Input: dimensioned drawing with shaded views. Units: mm. Origin: part minimum x, y, z. Give positions to 0.01 mm unless a question says otherwise; leave off trailing zeros. Loops run counter-clockwise (first coordinate to the right, second up) from the corner with the lowest first, then second, coordinate; pieces in that order, holes last. Notation, with made-up numbers: M 55.25,29.5 L 107.25,29.5 A18 ccw 107.25,44.5 Z; hole C 43.5,41 d5. An arc over 180 degrees is marked long. Answer in a Markdown table with one row per item.
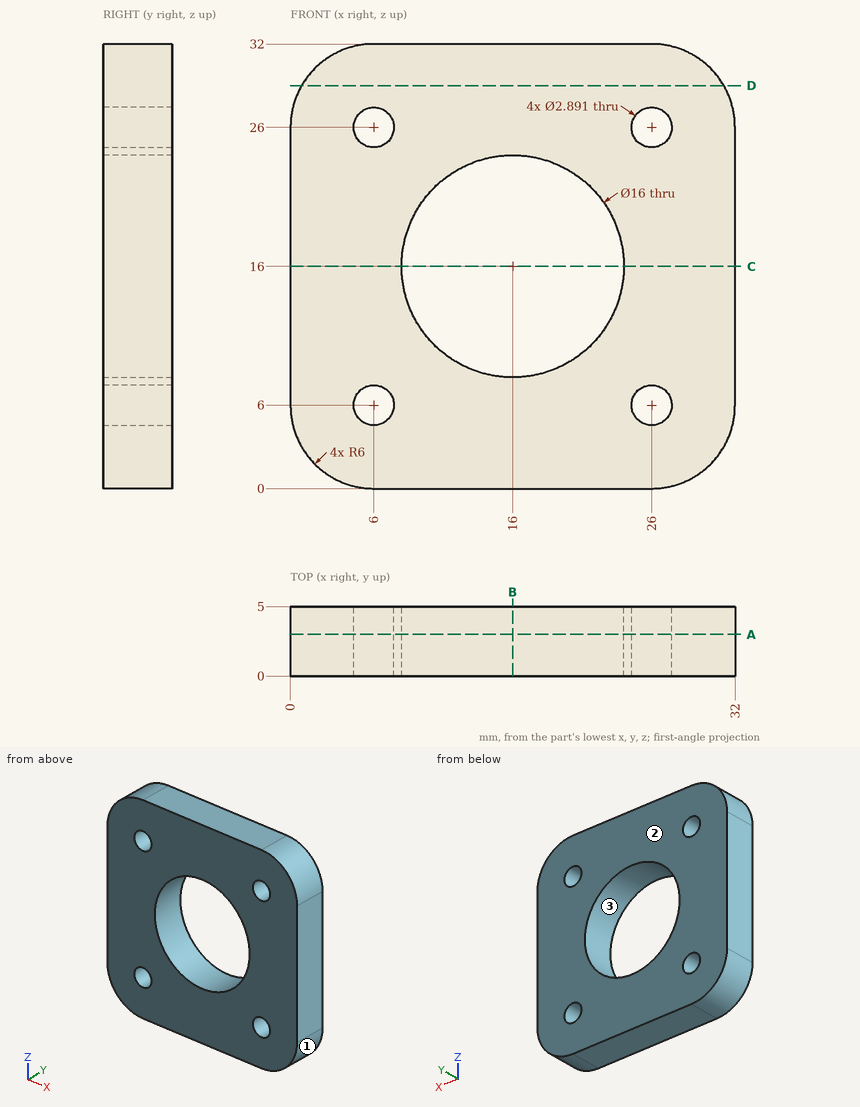
Q1. Section query A-A (y = 3). Output: boundary loops of the cut face in (x, z) (1 decimal), plus the area to 3 significant figures.
Values follow:
| item | result |
|---|---|
| outline | M 0,6 A6 ccw 6,0 L 26,0 A6 ccw 32,6 L 32,26 A6 ccw 26,32 L 6,32 A6 ccw 0,26 Z; hole C 6,6 d2.9; hole C 6,26 d2.9; hole C 16,16 d16; hole C 26,6 d2.9; hole C 26,26 d2.9 |
| area | 766 mm^2 |
Q2. Section query D-D (z = 29). Output: boundary loops of the cut face in (x, y), plus the area to 3 significant figures.
Values follow:
| item | result |
|---|---|
| outline | M 0.8,0 L 31.2,0 L 31.2,5 L 0.8,5 Z |
| area | 152 mm^2 |
Q3. Mould query, pull axis X, two halves, no side actions, for the marked faces 1, 2 and 3. Classes: +X half, -X half, draft (parallel to the pull), parting line (faces both ways), or undercut.
Values follow:
| item | result |
|---|---|
| face 1 | +X half |
| face 2 | draft |
| face 3 | undercut |
Q4. Section query B-B (x = 16). Output: boundary loops of the cut face in (y, z).
Values follow:
| item | result |
|---|---|
| outline | M 0,0 L 5,0 L 5,8 L 0,8 Z; M 0,24 L 5,24 L 5,32 L 0,32 Z |
Q5. Section query C-C (z = 16). Output: boundary loops of the cut face in (x, y), plus the area to 3 significant figures.
Values follow:
| item | result |
|---|---|
| outline | M 0,0 L 8,0 L 8,5 L 0,5 Z; M 24,0 L 32,0 L 32,5 L 24,5 Z |
| area | 80.0 mm^2 |
Q6. Ray query, probe 1 along X at (y, z) = (2.1, 26) (1 decimal); probe 2 along Z at (x, y) = (5, 0.8) (1 decimal). Return the intervals inside material, ascending. Write a range as from..to.
Values follow:
| item | result |
|---|---|
| probe 1 | 0..4.6, 7.4..24.6, 27.4..32 |
| probe 2 | 0.1..5, 7..25, 27..31.9 |
